Print and shaded views of the part. All mm, measured from the part's lowest x, y and z. Coordinates: 2 decimals unless noted, no trailing zeros. Loops run counter-clockwise (first coordinate to the right, second up) from the corner with the lowest first, then second, coordinate; pieces in that order, holes last.
1) Saw through at C-C, the plane z = 7. Write the cut outline in (x, y).
2) Saw through at B-B, the plane x = 2.5. Write the cut outline in (y, z), and give its area (3 significant figures).
3) Saw through at A-A, the plane y = 19.5. Write the cut outline in (x, z).
4) Wall check: line 1 along X through (y, z) = (29, 19); line 2 along Z through (x, y) = (3, 15); line 3 along Z through (x, y) = (17, 18.5) (1 decimal). Give the ranges that are in metal, low to high.
5) Two-plate mould, pull along X, no slides. Class the marked faces 1, 2, 3 and 4: +X half, -X half, draft (parallel to the pull), parting line (faces both ways), or undercut.
6) Pin check, flat tips, straight feed: pin 1 Ø0.6 at (y, z) = (9.5, 19) entering from -X; pin 2 Ø1.5 at (y, z) = (18, 19) entering from +X; pin 3 Ø2.5 at (y, z) = (15, 19.5) entering from -X. Stop position of each tip, or through.
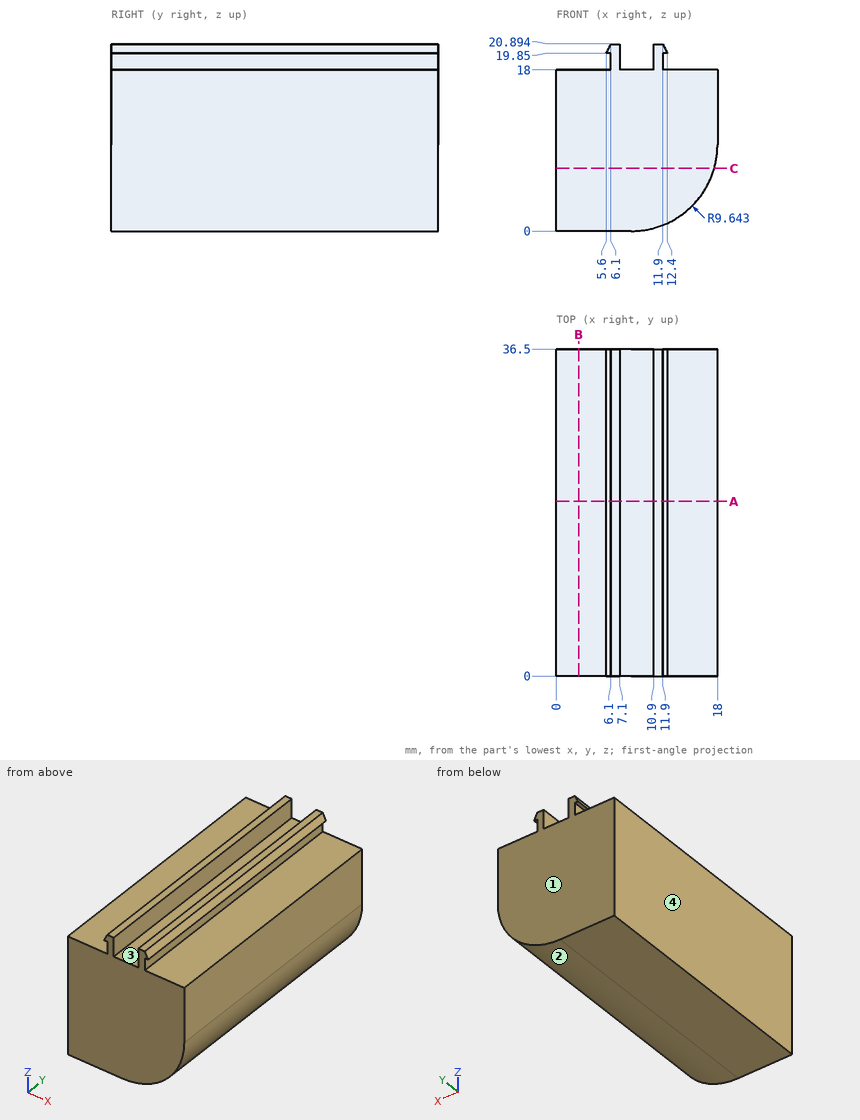
Data:
1. outline: (0, 0) - (17.63, 0) - (17.63, 36.5) - (0, 36.5) - close
2. outline: (0, 0) - (36.5, 0) - (36.5, 18) - (0, 18) - close
2. area: 657 mm2
3. outline: (0, 0) - (8.36, 0) arc R9.64 ccw to (18, 9.64) - (18, 18) - (11.9, 18) - (11.9, 19.85) - (12.4, 19.85) - (11.9, 20.89) - (10.9, 20.89) - (10.9, 18) - (7.1, 18) - (7.1, 20.89) - (6.1, 20.89) - (5.6, 19.85) - (6.1, 19.85) - (6.1, 18) - (0, 18) - close
4. line 1: x = 6.1 to 7.1, 10.9 to 11.9
4. line 2: z = 0 to 18
4. line 3: z = 5.4 to 18
5. face 1: draft
5. face 2: +X half
5. face 3: undercut
5. face 4: -X half
6. pin 1: stops at x = 6.1
6. pin 2: stops at x = 11.9
6. pin 3: stops at x = 5.6
